The listing builds one solid part. Answer for the finished solid, in the listing's coordinates (mm). A direction names the side the tool comes from. Round coordinates to 2 decimals unless told otherwise and drop trailing zeros. Write each loop counter-clockwise with the first axis right and the second up, starting at its lowest first coordinate (ties: lowest second). Pieces come first, ordered by that corner, then holes. Notation, with made-up numbers: (70, 27.25) - (106, 27.25) arc R25 ccw to (106, 40.25) - close; hole circle Ø9 at (67.25, -1). An arc over 180 degrees is marked (long way). Return JSON: item names as keys, results as strings. Group by question number.
from build123d import *

# Parameters (mm, degrees)
F0_W            = 25.4
F0_H            = 25.4
F1_DEPTH        = 1.27
F3_DEPTH        = 2.54
F2_R            = 3.4925
F4_DEPTH        = 2.54
F5_DEPTH        = 2.54
F5_COPIES_COUNT = 4
F7_DEPTH        = 2.541
F7_COPIES_COUNT = 4


# Not quite as in the source:
# - a pattern or mirror of a feature is missing from the dataset's text; its kind, count and spacing are read off the source's solid


with BuildPart() as f1:
    # F0 (on Top) → F1 (new body, symmetric)
    with BuildSketch(Plane.XY):
        Rectangle(F0_W, F0_H)
    extrude(amount=F1_DEPTH, both=True)

    # F2 (on face) → F3 (join)
    with BuildSketch(Plane.XY.offset(1.27)):
        Polygon((0, 10.1892549187), (-7.2048912482, 7.2048912482), (-10.1892549187, 0), (-7.2048912482, -7.2048912482), (0, -10.1892549187), (7.2048912482, -7.2048912482), (10.1892549187, 0), (7.2048912482, 7.2048912482), align=None)
        Polygon((-4.7748514527, 4.7748514527), (0, 6.7526596828), (4.7748514527, 4.7748514527), (6.7526596828, 0), (4.7748514527, -4.7748514527), (0, -6.7526596828), (-4.7748514527, -4.7748514527), (-6.7526596828, 0), align=None, mode=Mode.SUBTRACT)
    extrude(amount=F3_DEPTH)

    # F2 (on face) → F4 (join, through all)
    with BuildSketch(Plane.XY.offset(1.27)):
        Circle(F2_R)
    extrude(amount=F4_DEPTH)

    # F2 (on face) → F5 (join, through all)
    with BuildSketch(Plane.XY.offset(1.27)):
        Polygon((-2.2352, 12.7), (-12.7, 12.7), (-12.7, 2.2352), (-9.6349310438, 9.6349310438), align=None)
    f5 = extrude(amount=F5_DEPTH)

    # F5_copies: F5 ×4 about axis
    f5_copies_axis = Axis((0, 0, 0), (0, 0, 1))
    for i in range(1, F5_COPIES_COUNT):
        add(f5.rotate(f5_copies_axis, i * 360 / F5_COPIES_COUNT))

    # F6 (on face) → F7 (cut, through all)
    with BuildSketch(Plane.XY.offset(1.27)):
        Polygon((-8.6189310438, 10.0557720231), (-6.1888912482, 7.6257322276), (0, 10.1892549187), (6.1888912482, 7.6257322276), (8.6189310438, 10.0557720231), (2.2352, 12.7), (-2.2352, 12.7), align=None)
    f7 = extrude(amount=-F7_DEPTH, mode=Mode.SUBTRACT)

    # F7_copies: F7 ×4 about axis
    f7_copies_axis = Axis((0, 0, 0), (0, 0, 1))
    for i in range(1, F7_COPIES_COUNT):
        add(f7.rotate(f7_copies_axis, i * 360 / F7_COPIES_COUNT), mode=Mode.SUBTRACT)


solid = f1.part
(1) For faces 1 (the flat face through (2.42, -5.75, 2.52)), 2 (the flat face through (-8.824, 7.387, 0.018)), 3 (the flat face through (0, 0, -1.27)), determine the directions among +Z, -Z, +X, -X, +Y, -Y from which every point of the face is accessible in a straight line to the end or side of a thin tool.
(2) Find section C-C (y = -5.5). Write down the section's boundary in (x, z).
(3) Find section A-A (z = 3.45). State how many separate pieces and enclosed holes the cut face has, plus the area to 3 significant figures.
(4) Find section B-B (x = -11). Write down the section's boundary in (y, z).
(5) Consider line 1 (Y direction, x = -5.25, z = 1.05); line 2 (Y direction, x = -8.75, z = 2.25); line 3 (X direction, y = 1.5, z = 1.6). Determine where each line is inside the solid, lowest interval first.
(6) Flat-ended cylindrical pins translate along their axes: pin 1 (1.5 mm diameter, centred on y = 0, z = 3, fed in from -X); pin 2 (1.2 mm diameter, centred on x = 8, y = -9, fed in from +Z); pin 3 (5 mm diameter, centred on x = 9.5, y = -3.5, fed in from +Z). Find the tip coordinate at first contact, or state that the pin passes through.
(7) Determine the mould class of faces 4 (the flat face through (-8, -12.7, 1)), 5 (the flat face through (2.35, 5.78, 2.52)), 6 (the flat face through (10, -10, 3.81)), 7 (the flat face through (-8.858, -7.421, 0.018)) for opening direction Y: +Y half, -Y half, draft (parallel to the pull), parting line (faces both ways), or undercut.
(8) Find section D-D (x = -4.25). Write down the section's boundary in (y, z).
Check sheet entries:
{
 "1": {"face 1": "+Z", "face 2": "+Z, -Z", "face 3": "-Z, +X, -X, +Y, -Y"},
 "2": {"outline": "(-12.7, -1.27) - (-11.35, -1.27) - (-11.35, 3.81) - (-12.7, 3.81) - close; (-7.91, -1.27) - (7.91, -1.27) - (7.91, 3.81) - (3.02, 3.81) - (3.02, 1.27) - (-3.02, 1.27) - (-3.02, 3.81) - (-7.91, 3.81) - close; (11.35, -1.27) - (12.7, -1.27) - (12.7, 3.81) - (11.35, 3.81) - close"},
 "3": {"separate pieces": "6", "enclosed holes": "1", "area": "331 mm^2"},
 "4": {"outline": "(-12.7, -1.27) - (-6.34, -1.27) - (-6.34, 3.81) - (-12.7, 3.81) - close; (6.34, -1.27) - (12.7, -1.27) - (12.7, 3.81) - (6.34, 3.81) - close"},
 "5": {"line 1": "y = -12.7 to -11.45, -8.01 to 8.01, 11.45 to 12.7", "line 2": "y = -12.7 to -10, -3.47 to 3.47, 10 to 12.7", "line 3": "x = -9.57 to -6.13, -3.15 to 3.15, 6.13 to 9.57"},
 "6": {"pin 1": "stops at x = -10.19", "pin 2": "stops at z = 1.27", "pin 3": "stops at z = 3.81"},
 "7": {"face 4": "-Y half", "face 5": "undercut", "face 6": "draft", "face 7": "undercut"},
 "8": {"outline": "(-12.7, -1.27) - (-11.87, -1.27) - (-11.87, 3.81) - (-12.7, 3.81) - close; (-8.43, -1.27) - (8.43, -1.27) - (8.43, 3.81) - (4.99, 3.81) - (4.99, 1.27) - (-4.99, 1.27) - (-4.99, 3.81) - (-8.43, 3.81) - close; (11.87, -1.27) - (12.7, -1.27) - (12.7, 3.81) - (11.87, 3.81) - close"}
}
